Geometry: final body of the model. Coordinates: model frame, mm. A direction names the side the tool comes from. Give positions to 0.01 mm unless a question says otherwise; leave off trailing zeros. Write each loop counter-clockwise with the first axis right and the second up, starting at its lowest first coordinate (ties: lowest second). Pieces come first, ordered by that corner, then holes. Notation, with made-up numbers: M 60.5,60.5 L 96.5,60.5 A25 cw 96.5,72.5 Z; hole C 13,-27 d7. An arc over 180 degrees is marked long. Use one line per item in the form item = value. Start each with the question number.
Item 1: Section query B-B on x = 65.5. Return loops of the section in (y, z).
Item 2: Access query for faces 1 (the flat face through (-77.621, -134.164, 4.93)), 2 (the flat face through (77, 5, 5)), 3 (the flat face through (1, 1, 10)), 4 (the flat face through (-69.768, 135.771, 4.93)), 5 (the flat face through (-43.067, 64.594, 4.93)). Directions: +Z, -Z, +X, -X, +Y, -Y. A direction counts if a zero-diameter tool reaches every point of the face in a straight line with its end or side. Return the directions, or none.
Item 3: Pull-direction query (Y, two-part tool) for faces 6 (the flat face through (-69.74, -135.87, 4.93)), 7 (the flat face through (75, -5, 5)), 8 (the flat face through (-77.379, 134.304, 4.93)); classes: released by +Y, released by -Y, zero draft, split by the parting line, or undercut.
Item 4: Material intervals for line 1 along Y through (x, z) = (97.5, 6.5); line 2 along Y through (x, z) = (-8, 6.75); line 3 along Y through (x, z) = (-67.5, 3.75), sorted ascending. Write a range as from..to.
Item 5: Contact query for flat-ended pins moving along their axis: P1, Ø5, axis at x = 74, z = 5.5, coming from the +Y side; P2, Ø3, axis at y = 1.5, z = 5.5, coming from the -X side; P3, Ø8, axis at x = -55.5, y = 88.5, coming from the -Z side; P4, Ø4, axis at y = 47.5, z = 4.5, coming from the +X side. Output: stop coordinate, or through.
Item 6: Section query A-A on z = 6.75. Return loops of the section in (x, y).
Item 7: Section query C-C on y = -73. Return loops of the section in (x, z).
from build123d import *

# Parameters (mm, degrees)
BOSS_EXTRUDE1_DEPTH = 10
CIRPATTERN1_COUNT   = 3


with BuildPart() as part:
    # Sketch1 → Boss-Extrude1 (new body)
    with BuildSketch(Plane.XY):
        Polygon((155, 10), (150, 5), (0, 5), (0, -5), (150, -5), (155, -10), align=None)
    boss_extrude1 = extrude(amount=BOSS_EXTRUDE1_DEPTH)

    # CirPattern1: Boss-Extrude1 ×3 about axis
    cirpattern1_axis = Axis((0, 0, 0), (0, 0, 1))
    for i in range(1, CIRPATTERN1_COUNT):
        add(boss_extrude1.rotate(cirpattern1_axis, i * 360 / CIRPATTERN1_COUNT))


solid = part.part
Answer sheet:
q1.outline = M -5,0 L 5,0 L 5,10 L -5,10 Z
q2.face_1 = +Z, -Z, -X, -Y
q2.face_2 = +Z, -Z, +Y
q2.face_3 = +Z, +X, -X, +Y, -Y
q2.face_4 = +Z, -Z, +X
q2.face_5 = +Z, -Z, -X
q3.face_6 = undercut
q3.face_7 = released by -Y
q3.face_8 = released by +Y
q4.line_1 = -5..5
q4.line_2 = -23.86..-3.86, 3.86..23.86
q4.line_3 = -126.91..-106.91, 106.91..126.91
q5.P1 = 5
q5.P2 = -7.51
q5.P3 = 0
q5.P4 = -20.5
q6.outline = M -86.16,-129.23 L -68.84,-139.23 L -70.67,-132.4 L 2.89,-5 L 150,-5 L 155,-10 L 155,10 L 150,5 L 2.89,5 L -70.67,132.4 L -68.84,139.23 L -86.16,129.23 L -79.33,127.4 L -5.77,0 L -79.33,-127.4 Z
q7.outline = M -47.92,0 L -36.37,0 L -36.37,10 L -47.92,10 Z
